```python
from build123d import *

# Parameters (mm, degrees)
SKETCH1_W           = 50
SKETCH1_H           = 100
BOSS_EXTRUDE1_DEPTH = 25


with BuildPart() as part:
    # Sketch1 → Boss-Extrude1 (new body)
    with BuildSketch(Plane(origin=(0, 0, 0), x_dir=(1, 0, 0), z_dir=(0, 1, 0))):
        Polygon((-457.962648343, 1946.847529943), (-457.962648343, -53.152470057), (342.037351657, -53.152470057), (342.037351657, 1946.847529943), (-32.962648343, 1946.847529943), (-32.962648343, 1846.847529943), (-82.962648343, 1846.847529943), (-82.962648343, 1946.847529943), align=None)
        with Locations((-57.962648343, 1696.847529943)):
            Rectangle(SKETCH1_W, SKETCH1_H, mode=Mode.SUBTRACT)
        with Locations((-57.962648343, 1496.847529943)):
            Rectangle(SKETCH1_W, SKETCH1_H, mode=Mode.SUBTRACT)
        with Locations((-57.962648343, 1296.847529943)):
            Rectangle(SKETCH1_W, SKETCH1_H, mode=Mode.SUBTRACT)
        with Locations((-57.962648343, 1096.847529943)):
            Rectangle(SKETCH1_W, SKETCH1_H, mode=Mode.SUBTRACT)
        with Locations((-57.962648343, 896.847529943)):
            Rectangle(SKETCH1_W, SKETCH1_H, mode=Mode.SUBTRACT)
        with Locations((-57.962648343, 696.847529943)):
            Rectangle(SKETCH1_W, SKETCH1_H, mode=Mode.SUBTRACT)
        with Locations((-57.962648343, 496.847529943)):
            Rectangle(SKETCH1_W, SKETCH1_H, mode=Mode.SUBTRACT)
        with Locations((-57.962648343, 296.847529943)):
            Rectangle(SKETCH1_W, SKETCH1_H, mode=Mode.SUBTRACT)
        with Locations((-57.962648343, 96.847529943)):
            Rectangle(SKETCH1_W, SKETCH1_H, mode=Mode.SUBTRACT)
    extrude(amount=BOSS_EXTRUDE1_DEPTH)


solid = part.part
```
Work out the finished part from the listing and answer in its coordinate system (mm). Coordinates: 2 decimals unless noted, no trailing zeros. Loops run counter-clockwise (first coordinate to the right, second up) from the corner with the lowest first, then second, coordinate; pieces in that order, holes last.
1) Section A-A (z = -269.5) is taken. Give the vertices of the cut face in (x, y).
Results:
outline: (-457.96, 0) - (-82.96, 0) - (-82.96, 25) - (-457.96, 25) - close; (-32.96, 0) - (342.04, 0) - (342.04, 25) - (-32.96, 25) - close
2) Section B-B (y = 10.75) is taken. Give the number of separate pieces and of enclosed holes in the cut face, plus the area to 3 significant figures.
Results:
separate pieces: 1
enclosed holes: 9
area: 1,550,000 mm2
3) A flat-ended cylindrical pin translates along its axis: pin 1 (12.5 mm diameter, centred on x = -61, y = 13, fed in from -Z). Find the tip coordinate at first contact, or state that the pin passes through.
Results:
pin 1: stops at z = -1846.85
4) Consider probe 1 along X at (y, z) = (19.5, -332). Determine where the line is inside the solid, lowest interval first.
Results:
probe 1: x = -457.96 to -82.96, -32.96 to 342.04
